Solid Edge part; units mm, degrees
sketch "Sketch1" plane through (0, 0, 0) normal (0, 0, 1) x (1, 0, 0)
  circle A0 centre (0, 0) radius 4
extrude "Protrusion1" add sketch "Sketch1" along normal blind 43.5
hole "Hole_3" at (0, 0, 0) direction (0, 0, 1) diameter 3.242 depth 10 thread major 4 thread length 8
hole "Hole_4" at (0, 0, 43.5) direction (0, 0, -1) diameter 3.242 depth 10 thread major 4 thread length 8
Source: CAD feature listing. Evaluate the final solid. Frame: model axes, mm. A direction names the side the tool comes from. Give positions to 0.01 mm unless a question says otherwise; leave off trailing zeros. Write each loop counter-clockwise with the first axis right and the second up, starting at its lowest first coordinate (ties: lowest second). Pieces come first, ordered by that corner, then holes.
1. First-contact query: pin 1 (1 mm diameter, centred on x = -0.5, y = -0.5, fed in from -Z); pin 2 (2.5 mm diameter, centred on x = 0, y = 0, fed in from +Z); pin 3 (1 mm diameter, centred on y = 3, z = 5, fed in from -X). Flat tips, straight axial feed; report the tip coordinate or a pass-through.
2. Access query for faces 5 (the face through (1.438, -0.748, 38.43)), 6 (the face through (0, 0, 10)), 7 (the face through (2, 0, 0)). Directions: +Z, -Z, +X, -X, +Y, -Y. A direction counts if a zero-diameter tool reaches every point of the face in a straight line with its end or side. Return the directions, or none.
3. Section query C-C (z = 31). Return the cut outline in (x, y), then the cut area to 3 significant figures.
4. Section query D-D (z = 4). Return the cut outline in (x, y).
5. Pull-direction query (Y, two-part tool) for faces 1 (the face through (2, 0, 43.5)), 2 (the face through (1.438, 0.748, 5.07)), 3 (the face through (-0.867, 3.905, 21.446)), 4 (the face through (0, 0, 33.5)); classes: +Y half, -Y half, draft (parallel to the pull), parting line (faces both ways), or undercut.
6. Material intervals for line 1 along Y through (x, z) = (0, 41.5); line 2 along Z through (x, y) = (-0.25, -0.5); line 3 along X through (y, z) = (1, 34), sorted ascending.
7. Section query A-A (y = 0). Return the cut outline in (x, z), then the cut area to 3 significant figures.
Output values:
1. pin 1: stops at z = 10
1. pin 2: stops at z = 33.5
1. pin 3: stops at x = -3.12
2. face 5: +Z
2. face 6: -Z
2. face 7: -Z, +X, -X, +Y, -Y
3. outline: circle Ø8 at (0, 0)
3. area: 50.3 mm2
4. outline: circle Ø8 at (0, 0); hole circle Ø3.24 at (0, 0)
5. face 1: draft
5. face 2: undercut
5. face 3: parting line
5. face 4: undercut
6. line 1: y = -4 to -1.62, 1.62 to 4
6. line 2: z = 10 to 33.5
6. line 3: x = -3.87 to -1.28, 1.28 to 3.87
7. outline: (-4, 0) - (-1.62, 0) - (-1.62, 10) - (1.62, 10) - (1.62, 0) - (4, 0) - (4, 43.5) - (1.62, 43.5) - (1.62, 33.5) - (-1.62, 33.5) - (-1.62, 43.5) - (-4, 43.5) - close
7. area: 283 mm2
